Input: dimensioned drawing with shaded views. Units: mm. Origin: part minimum x, y, z. A direction names the side the tool comes from. Round coordinates to 2 decimals unless told otherwise and drop trailing zeros. Order: outer loops, then holes, each group sorted by start corner. A loop starts at its lowest first (then second) coordinate and runs counter-clockwise, first axis right, second up. Notation, with made-up numbers: M 85.25,-11.75 L 110.25,-11.75 A6 cw 110.25,-1.75 Z; hole C 80,-2.75 d5. An arc over 180 degrees is marked long. One line per question, with ' | ' between items.
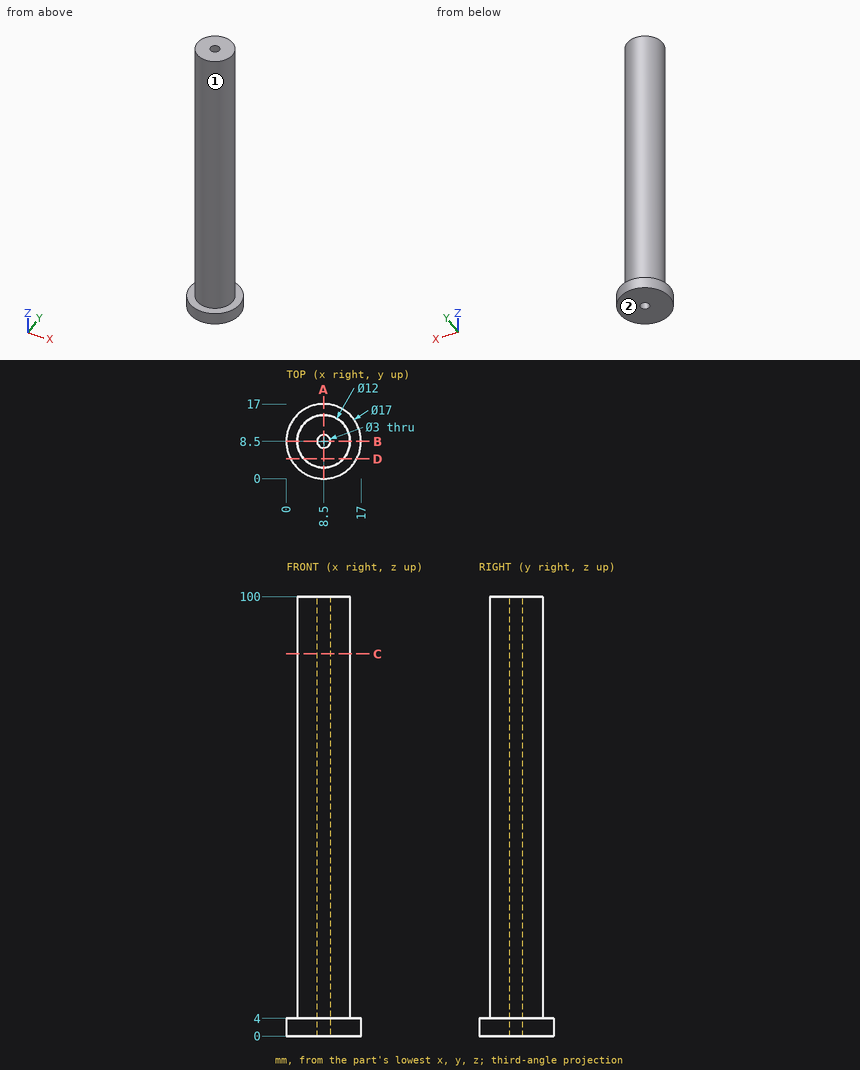
Item 1: Line query: line 1 along Y through (x, z) = (8.5, 24); line 2 along Z through (x, y) = (12.25, 15.75); line 3 along Y through (x, z) = (9.5, 39.5). Output: solid intervals per line, ascending. Write a range as from..to.
Report:
line 1: 2.5..7, 10..14.5 | line 2: 0..4 | line 3: 2.58..7.38, 9.62..14.42
Item 2: First-contact query: pin 1 (3 mm diameter, centred on x = 15, y = 12.5, fed in from +Z); pin 2 (3 mm diameter, centred on x = 8.5, z = 37, fed in from +Y); pin 3 (1 mm diameter, centred on y = 4, z = 27.5, fed in from +X). Flat tips, straight axial feed; report the tip coordinate or a pass-through.
Report:
pin 1: z = 4 | pin 2: y = 14.5 | pin 3: x = 12.97
Item 3: Access query for the marked faces 1 and 2. Directions: +Z, -Z, +X, -X, +Y, -Y. A direction counts if a zero-diameter tool reaches every point of the face in a straight line with its end or side. Return the directions, or none.
Report:
face 1: +Z | face 2: -Z, +X, -X, +Y, -Y
Item 4: Section query C-C, the plane z = 87. Return loops of the section in (x, y), plus the area to 3 significant figures.
Report:
outline: C 8.5,8.5 d12; hole C 8.5,8.5 d3 | area: 106 mm²
Item 5: Section query A-A, the plane x = 8.5. Return loops of the section in (y, z).
Report:
outline: M 0,0 L 7,0 L 7,100 L 2.5,100 L 2.5,4 L 0,4 Z; M 10,0 L 17,0 L 17,4 L 14.5,4 L 14.5,100 L 10,100 Z
Item 6: Section query D-D, the plane y = 4.5. Return loops of the section in (x, z), plus the area to 3 significant figures.
Report:
outline: M 1,0 L 16,0 L 16,4 L 12.97,4 L 12.97,100 L 4.03,100 L 4.03,4 L 1,4 Z | area: 919 mm²
